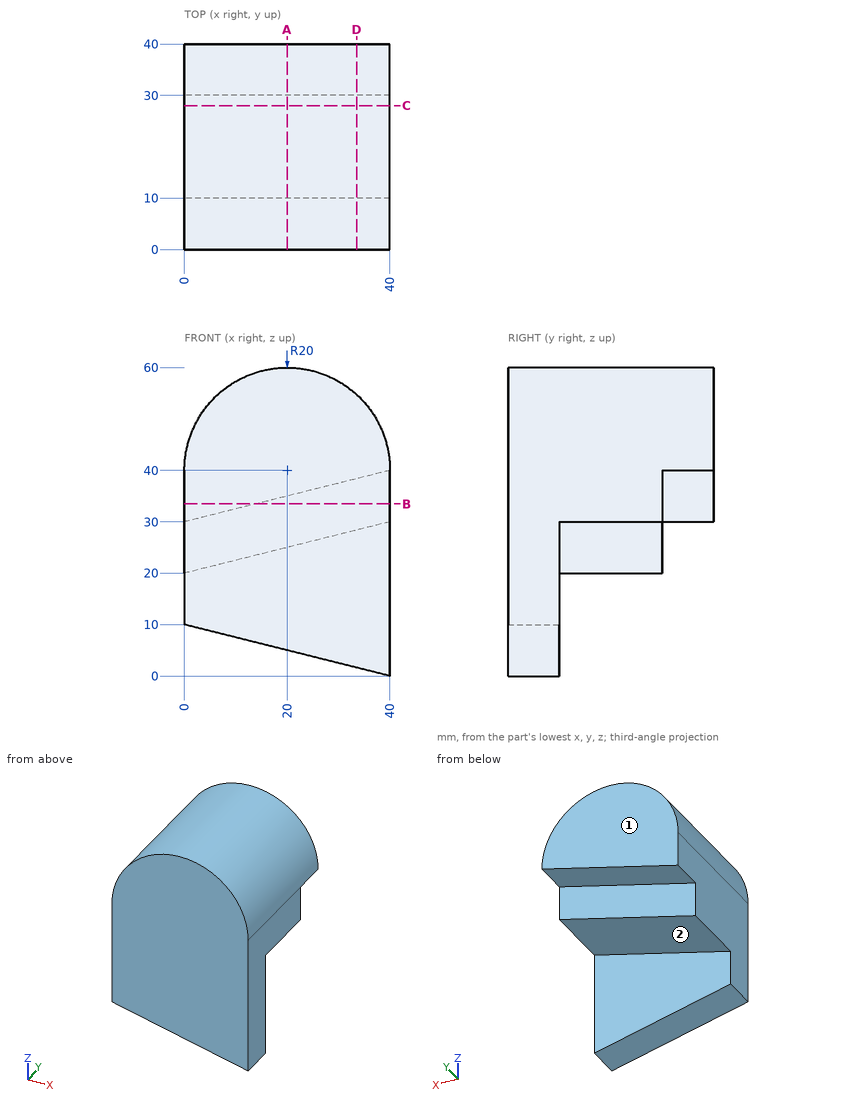
Geometry: see drawing. Coordinates: mm, zero at the bounding-box minimum. A direction names the side the tool comes from. Round coordinates to 2 decimals unless told otherwise and drop trailing zeros. Write each loop counter-clockwise with the first axis right and the second up, starting at its lowest first coordinate (ties: lowest second). Pieces come first, ordered by that corner, then holes.
1) Cut plane B-B (z = 33.5). Return the cut outline in (x, y), then the cut area to 3 significant figures.
2) Contact query for flat-ended pins moving along their axis: P1, Ø6, axis at x = 8, y = 10.5, coming from the -Z side; P2, Ø8, axis at x = 26, z = 24, coming from the +Y side; P3, Ø12, axis at x = 24.5, y = 24, coming from the -Z side (3 decimals); P4, Ø6, axis at x = 34, z = 39, coming from the -Y side. Output: stop coordinate, or through.
3) Cut plane A-A (x = 20). Return the cut outline in (y, z), then the cut area to 3 significant figures.
4) Cut plane C-C (y = 28). Return the cut outline in (x, z).
5) Ray query, L1, parallel to Y at x = 6.5, z = 23; L2, parallel to Y at x = 38.5, z = 14.5; L3, parallel to X at y = 16, z = 40.5. Return the intervals inside material, ascending.
6) Reachability of the marked faces 1 and 2 from +Z, -Z, +X, -X, +Y, -Y: full face, straight path, thin tool, end or side. Return the list, or none.
7) Cut plane D-D (x = 33.5). Return the cut outline in (y, z) (3 decimals), then the cut area to 3 significant figures.
Geometry says:
1. outline: (0, 0) - (40, 0) - (40, 30) - (14, 30) - (14, 40) - (0, 40) - close
1. area: 1,340 mm2
2. P1: stops at z = 7.26
2. P2: stops at y = 30
2. P3: stops at z = 24.625
2. P4: stops at y = 0
3. outline: (0, 5) - (10, 5) - (10, 25) - (30, 25) - (30, 35) - (40, 35) - (40, 60) - (0, 60) - close
3. area: 1,500 mm2
4. outline: (0, 20) - (40, 30) - (40, 40) arc R20 ccw to (0, 40) - close
5. L1: y = 0 to 30
5. L2: y = 0 to 10
5. L3: x = 0.01 to 39.99
6. face 1: +Z, -Z, +X, -X, +Y
6. face 2: -Z, +X, +Y
7. outline: (0, 1.625) - (10, 1.625) - (10, 28.375) - (30, 28.375) - (30, 38.375) - (40, 38.375) - (40, 54.756) - (0, 54.756) - close
7. area: 1,220 mm2
